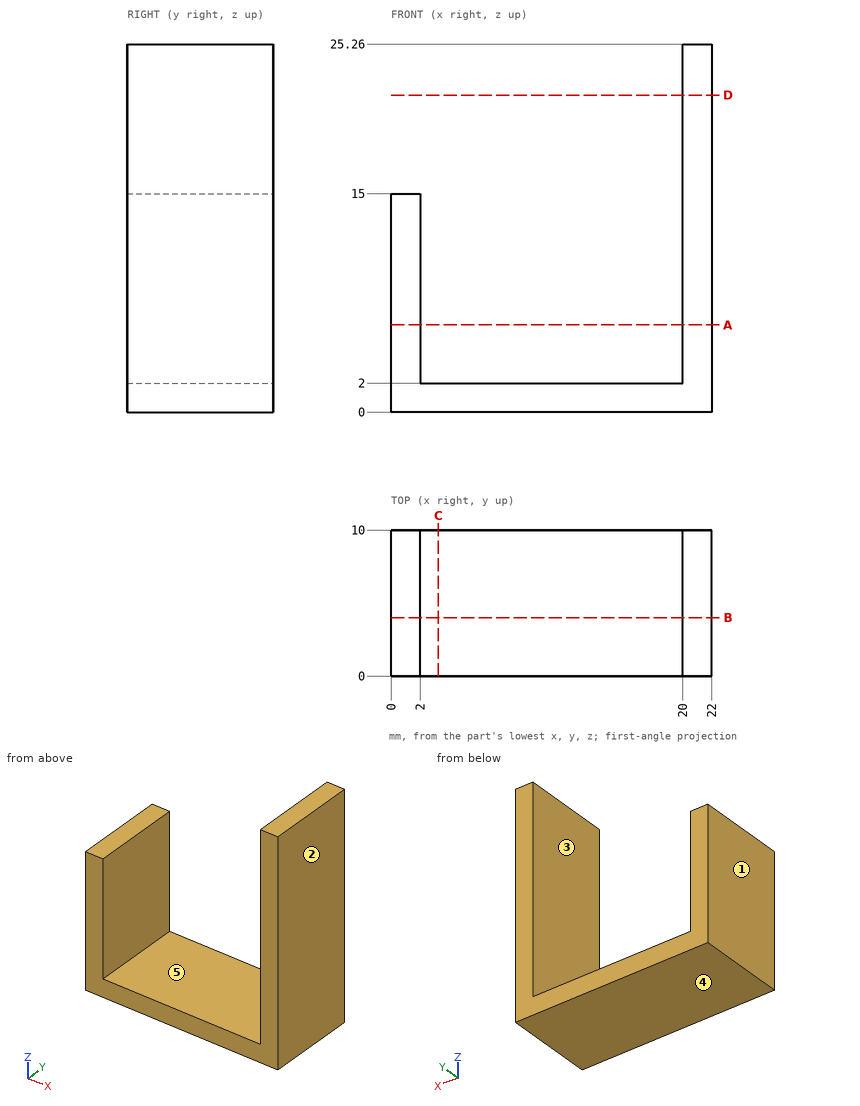
Study the drawing (mm; zero at the part's minimum x, y, z) and answer. A direction names the side the tool comes from. Coordinates: 2 decimals unless noted, no trailing zeros. Loops run counter-clockwise (first coordinate to the right, second up) from the corner with the lowest first, then second, coordinate; pieces in that order, holes last. Notation, with made-up numbers: (6.5, 52.25) -> (56.5, 52.25) arc R29 ccw to (56.5, 90.25) -> close; hole circle Ø3 at (32.5, -7.75). An arc over 180 degrees is marked (long way). Answer in a Markdown table with one row per item. Add a question column.
1. The part is cut by section A-A, the plane z = 6. Write down the section's boundary in (x, y), then the cut area to 3 significant figures.
2. The part is cut by section D-D, the plane z = 21.75. Write down the section's boundary in (x, y).
3. For the marked faces 4 and 5, determine the directions among +Z, -Z, +X, -X, +Y, -Y from which every point of the face is accessible in a straight line to the end or side of a thin tool.
4. The part is cut by section B-B, the plane y = 4. Write down the section's boundary in (x, z).
5. The part is cut by section C-C, the plane x = 3.25. Write down the section's boundary in (y, z).
6. Determine the mould class of the marked faces 1, 2 and 3 for opening direction X: +X half, -X half, draft (parallel to the pull), parting line (faces both ways), or undercut.
7. Flat-ended cylindrical pins translate along their axes: P1, Ø5, axis at x = 3, y = 1.5, coming from the +Z side; P2, Ø2, axis at y = 3, z = 18.5, coming from the -X side; P3, Ø1.5, axis at x = 3.5, y = 7.5, coming from the +Z side. Find the tip coordinate at first contact, or state that the pin passes through.
8. Consider line 1 (X direction, y = 6.25, z = 5.25); line 2 (Z direction, x = 10.5, y = 6); line 3 (X direction, y = 9, z = 18.75). Determine where each line is inside the solid, lowest interval first. Write a range as [from, to].
Answer below:
| question | item | result |
|---|---|---|
| 1 | outline | (0, 0) -> (2, 0) -> (2, 10) -> (0, 10) -> close; (20, 0) -> (22, 0) -> (22, 10) -> (20, 10) -> close |
| 1 | area | 40.0 mm2 |
| 2 | outline | (20, 0) -> (22, 0) -> (22, 10) -> (20, 10) -> close |
| 3 | face 4 | -Z, +X, -X, +Y, -Y |
| 3 | face 5 | +Z, +Y, -Y |
| 4 | outline | (0, 0) -> (22, 0) -> (22, 25.26) -> (20, 25.26) -> (20, 2) -> (2, 2) -> (2, 15) -> (0, 15) -> close |
| 5 | outline | (0, 0) -> (10, 0) -> (10, 2) -> (0, 2) -> close |
| 6 | face 1 | -X half |
| 6 | face 2 | +X half |
| 6 | face 3 | undercut |
| 7 | P1 | z = 15 |
| 7 | P2 | x = 20 |
| 7 | P3 | z = 2 |
| 8 | line 1 | [0, 2], [20, 22] |
| 8 | line 2 | [0, 2] |
| 8 | line 3 | [20, 22] |
